Could you check a few things on this model? Use its own coordinates, in mm. A direction names the side the tool comes from. Round coordinates to 2 decimals unless told otherwise and drop trailing zeros. Order: outer loops, then holes, each group sorted by start corner. A loop starts at its lowest first (then second) coordinate and runs counter-clockwise, first axis right, second up. Notation, with made-up numbers: M -14,24.25 L 35,24.25 A22 cw 35,37.25 Z; hole C -36,-10 d3. An arc over 180 degrees is marked long. Write each question's results on one line, items separated by ' | '. Start each with the question number.
1. Please list where these lines run through material, in increasing order: L1, parallel to Z at x = -729.5, y = -79; L2, parallel to Y at x = -164.5, z = 859.5; L3, parallel to Z at x = 705, y = 2.
2. Suppose I cut it at D-D on y = -146.5. Write out the boundary of the cut face in (x, z).
3. Suppose I cut it at C-C on z = 328.5. Write out the boundary of the cut face in (x, y), and give its area (3 significant figures).
4. Suppose I cut it at B-B on x = -156. Write out the boundary of the cut face in (y, z), and give its area (3 significant figures).
5. Suppose I cut it at A-A on y = 96. Write out the boundary of the cut face in (x, z).
6. For faces 1 (the flat face through (0, -225, 1141)), 2 (the flat face through (-12, 25, 475)), which set-ups out of +Z, -Z, +X, -X, +Y, -Y let a thin tool reach every point of the face, with its end or its side?
7. I'm going to push flat-ended pins straight in: pin 1 (1.5 mm diameter, centred on y = 3, z = 494.5, fed in from -X); pin 2 (12 mm diameter, centred on x = 166, y = -84, fed in from +Z); pin 3 (5 mm diameter, centred on x = 32, z = 93.5, fed in from +Y). Where does each tip first touch, or does it pass through?
from build123d import *

# Parameters (mm, degrees)
F1_DEPTH   = 25
F3_DEPTH   = 200
F4_W       = 1734.5163099376
F4_H       = 100
F1_FACE1_W = 1734.5163099376
F1_FACE1_H = 50
F5_DEPTH   = 50


with BuildPart() as f1:
    # F0 (on Front) → F1 (new body, symmetric)
    with BuildSketch(Plane.XZ):
        Polygon((0, 1200), (-867.2581549688, 0), (867.2581549688, 0), align=None)
    extrude(amount=F1_DEPTH, both=True)

    # F2 (on face) → F3 (join)
    with BuildSketch(Plane.XZ.offset(25)):
        with BuildLine():
            ThreePointArc((-28.3671346864, 1160.7492170254), (-10.7738174752, 1106.9473358987), (35, 1140.2478592731))
            ThreePointArc((35, 1140.2478592731), (33.3005233016, 1151.0216769733), (28.3671344093, 1160.7492174087))
            ThreePointArc((28.3671344093, 1160.7492174087), (-2.365e-07, 1175.2478592731), (-28.3671346864, 1160.7492170254))
        make_face()
    extrude(amount=F3_DEPTH)

    # F4 (on face) + F1_face1 (on face) → F5 (join)
    with BuildSketch(Plane(origin=(0, 0, 0), x_dir=(1, 0, 0), z_dir=(0, 0, -1))):
        with Locations((0, 75)):
            Rectangle(F4_W, F4_H)
        with Locations((0, -75)):
            Rectangle(F4_W, F4_H)
    with BuildSketch(Plane(origin=(0, 0, 0), x_dir=(1, 0, 0), z_dir=(0, 0, -1))):
        Rectangle(F1_FACE1_W, F1_FACE1_H)
    extrude(amount=F5_DEPTH)


solid = f1.part
Filled sheet:
1) L1: z = -50 to 0 | L2: y = -25 to 25 | L3: z = -50 to 224.51
2) outline: C 0,1140.25 d70
3) outline: M -629.85,-25 L 629.85,-25 L 629.85,25 L -629.85,25 Z | area: 63,000 mm^2
4) outline: M -125,-50 L 125,-50 L 125,0 L 25,0 L 25,984.15 L -25,984.15 L -25,0 L -125,0 Z | area: 61,700 mm^2
5) outline: M -867.26,-50 L 867.26,-50 L 867.26,0 L -867.26,0 Z
6) face 1: +Z, -Z, +X, -X, -Y | face 2: +Z, +X, -X, +Y
7) pin 1: stops at x = -510.42 | pin 2: stops at z = 0 | pin 3: stops at y = 25
